Autodesk Inventor part; units mm, degrees
ref_plane "YZ Plane" through (0, 0, 0) normal (1, 0, 0) x (0, 1, 0)
ref_plane "XZ Plane" through (0, 0, 0) normal (0, 1, 0) x (-1, 0, 0)
ref_plane "XY Plane" through (0, 0, 0) normal (0, 0, 1) x (1, 0, 0)
sketch "Schizzo2" plane through (0, 0, 0) normal (0, 1, 0) x (-1, 0, 0)
  line L0 (11.5, 11.5) -> (-11.5, 11.5)
  line L1 (-11.5, 11.5) -> (-11.5, -11.5)
  line L2 (-11.5, -11.5) -> (11.5, -11.5)
  line L3 (11.5, -11.5) -> (11.5, 11.5)
  line L4 (17.5, 17.5) -> (-17.5, 17.5)
  line L5 (-17.5, 17.5) -> (-17.5, -17.5)
  line L6 (-17.5, -17.5) -> (17.5, -17.5)
  line L7 (17.5, -17.5) -> (17.5, 17.5)
  line L8 (0, 0) -> (13.1636, 0) construction
  line L9 (0, 0) -> (0, -15.8245) construction
  line L10 (14.5, 14.5) -> (-14.5, 14.5)
  line L11 (-14.5, 14.5) -> (-14.5, -14.5)
  line L12 (-14.5, -14.5) -> (14.5, -14.5)
  line L13 (14.5, -14.5) -> (14.5, 14.5)
  dimension "d1" = 23
  dimension "d2" = 35
  dimension "d3" = 3
extrude "Estrusione1" add sketch "Schizzo2" along normal blind 10 and the other way blind 5 contours L13 L12 L11 L10
extrude "Estrusione2" add sketch "Schizzo2" against normal blind 90 contours L7 L6 L5 L4
extrude "Estrusione3" add sketch "Schizzo2" against normal blind 5 contours L3 L2 L1 L0
fillet "Raccordo1" radius 5 4 edges at (17.5, -45, 17.5) (17.5, -45, -17.5) (-17.5, -45, 17.5) (-17.5, -45, -17.5)
sketch "Schizzo3" plane through (0, 0, 0) normal (0, 0, 1) x (1, 0, 0)
  line L0 (-14.5, -5) -> (-14.5, 10)
  line L1 (-12.5, 0) -> (12.5, 0)
  line L2 (14.5, 10) -> (14.5, -5)
  line L3 (-14.5, 10) -> (14.5, 10)
  line L4 (0, 0) -> (0, 15.5409) construction
  line L5 (0, 0) -> (22.1267, 0) construction
  circle A0 centre (0, 5) radius 2.5
  dimension "d11" = 5
  dimension "d12" = 5
extrude "Estrusione4" cut sketch "Schizzo3" along normal through all both and the other way through all
sketch "Schizzo4" plane through (0, 0, 0) normal (1, 0, 0) x (0, 1, 0)
  line L0 (0, 12.5) -> (0, -12.5)
  line L1 (-90, -17.5) -> (0, -17.5)
  line L2 (0, 17.5) -> (-90, 17.5)
  line L3 (-90, -12.5) -> (-90, 12.5)
  line L4 (0, 0) -> (-112.8212, 0) construction
  line L5 (0, 0) -> (0, -73.2961) construction
  line L6 (-10, 10) -> (-20, 10)
  line L7 (-20, 10) -> (-20, -10)
  line L8 (-20, -10) -> (-10, -10)
  line L9 (-10, -10) -> (-10, 10)
  line L10 (-10, 5) -> (-20, 5)
  line L11 (-20, 5) -> (-20, -5)
  line L12 (-20, -5) -> (-10, -5)
  line L13 (-10, -5) -> (-10, 5)
  dimension "d17" = 10
  dimension "d18" = 20
  dimension "d19" = 10
  dimension "d20" = 10
extrude "Estrusione5" cut sketch "Schizzo4" along normal through all contours L9 L12 L7 L10
extrude "Estrusione6" add sketch "Schizzo4" along normal blind 27.5 contours L9 L10 L7 L6 | L9 L8 L7 L12
extrude "Estrusione7" cut sketch "Schizzo4" along normal up to surface (14.5 mm away) contours L9 L10 L7 L6 | L9 L8 L7 L12
properties part number "manico"
The listing builds one solid part. Answer for the finished solid, in the listing's coordinates (mm). A direction names the side the tool comes from. Give positions to 0.01 mm unless a question says otherwise; leave off trailing zeros. Write each loop counter-clockwise with the first axis right and the second up, starting at its lowest first coordinate (ties: lowest second). Pieces come first, ordered by that corner, then holes. Notation, with made-up numbers: (86.25, 56.5) -> (98.25, 56.5) arc R29 ccw to (98.25, 80.5) -> close; hole circle Ø1 at (3.5, -34.75). An arc over 180 degrees is marked (long way). Write item = value, one per line. Start each with the question number.
1) The part is cut by section C-C, the plane x = 0. Determine the outline of the cut face in (y, z).
2) Which of the six approach directions +Z, -Z, +X, -X, +Y, -Y give full straight-line access (tool end or side, diameter ignored) to faces 1 (the face through (-3, 5, 11.5)), 2 (the face through (22, -15, -10)), 3 (the face through (22, -10, -8)), 4 (the face through (21, -15, 5)), 5 (the face through (0, -47, -14.5))?
3) The part is cut by section B-B, the plane y = 5. Determine the outline of the cut face in (x, z), and give its area (3 significant figures).
4) The part is cut by section D-D, the plane y = -23. Determine the outline of the cut face in (x, z).
5) The part is cut by section A-A, the plane z = -2. Determine the outline of the cut face in (x, y), and give its area (3 significant figures).
6) Determine the mould class of faces 6 (the face through (16, 0, 0)), 7 (the face through (-14.5, -47, 0)), 8 (the face through (0, -44, 17.5)), 9 (the face through (11.5, 5, 0)) for opening direction Z: +Z half, -Z half, draft (parallel to the pull), parting line (faces both ways), or undercut.
7) Straight lines are drawn through the part: line 1 along Y through (x, z) = (17, -1.5); line 2 along Y through (x, z) = (0, 12.5); line 3 along Z through (x, y) = (11.5, -59). For each, find the intervals that lie inside material, in ascending order.
8) Each of these flat-tipped pins is pushed along its axis until it touches: pin 1 (4.5 mm diameter, centred on x = 0, y = 5, fed in from +Z); pin 2 (5.5 mm diameter, centred on x = 23, z = -7.5, fed in from +Y); pin 3 (8.5 mm diameter, centred on x = -3, z = 1.5, fed in from -Y); pin 4 (1 mm diameter, centred on y = -25, z = -1, fed in from +X). Where does it stop, or does it pass through?
Solutions:
q1.outline = (-90, -17.5) -> (0, -17.5) -> (0, -14.5) -> (2.5, -14.5) -> (2.5, -11.5) -> (0, -11.5) -> (0, 11.5) -> (2.5, 11.5) -> (2.5, 14.5) -> (0, 14.5) -> (0, 17.5) -> (-90, 17.5) -> (-90, 14.5) -> (-5, 14.5) -> (-5, -14.5) -> (-90, -14.5) -> close; (7.5, -14.5) -> (10, -14.5) -> (10, -11.5) -> (7.5, -11.5) -> close; (7.5, 11.5) -> (10, 11.5) -> (10, 14.5) -> (7.5, 14.5) -> close
q2.face_1 = +Y
q2.face_2 = -Z, +X, +Y, -Y
q2.face_3 = +Z, -Z, +X, +Y
q2.face_4 = +X
q2.face_5 = -Y
q3.outline = (-14.5, -14.5) -> (-2.5, -14.5) -> (-2.5, -11.5) -> (-11.5, -11.5) -> (-11.5, 11.5) -> (-2.5, 11.5) -> (-2.5, 14.5) -> (-14.5, 14.5) -> close; (2.5, -14.5) -> (14.5, -14.5) -> (14.5, 14.5) -> (2.5, 14.5) -> (2.5, 11.5) -> (11.5, 11.5) -> (11.5, -11.5) -> (2.5, -11.5) -> close
q3.area = 282 mm²
q4.outline = (-17.5, -12.5) arc R5 ccw to (-12.5, -17.5) -> (12.5, -17.5) arc R5 ccw to (17.5, -12.5) -> (17.5, 12.5) arc R5 ccw to (12.5, 17.5) -> (-12.5, 17.5) arc R5 ccw to (-17.5, 12.5) -> close; hole (-14.5, -14.5) -> (14.5, -14.5) -> (14.5, 14.5) -> (-14.5, 14.5) -> close
q5.outline = (-17.5, -90) -> (-14.5, -90) -> (-14.5, -5) -> (14.5, -5) -> (14.5, -10) -> (17.5, -10) -> (17.5, 0) -> (14.5, 0) -> (14.5, 10) -> (11.5, 10) -> (11.5, 0) -> (-11.5, 0) -> (-11.5, 10) -> (-14.5, 10) -> (-14.5, 0) -> (-17.5, 0) -> close; (14.5, -90) -> (17.5, -90) -> (17.5, -20) -> (14.5, -20) -> close
q5.area = 715 mm²
q6.face_6 = draft
q6.face_7 = undercut
q6.face_8 = +Z half
q6.face_9 = undercut
q7.line_1 = -90 to -20, -10 to 0
q7.line_2 = -5 to 2.5, 7.5 to 10
q7.line_3 = -17.5 to -14.5, 14.5 to 17.5
q8.pin_1 = through
q8.pin_2 = -10
q8.pin_3 = -5
q8.pin_4 = 17.5
